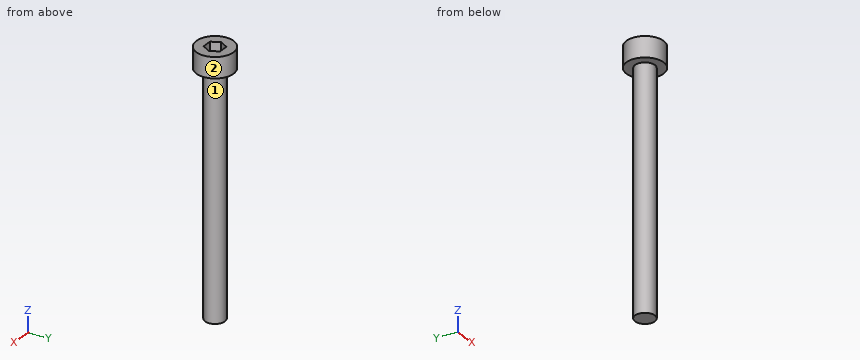
Solid Edge part; units mm, degrees
sketch "Sketch1" plane through (0, 0, 0) normal (0, 0, 1) x (1, 0, 0)
  circle A0 centre (0, 0) radius 2.725
extrude "Protrusion1" add sketch "Sketch1" against normal blind 3
sketch "Sketch2" plane through (0, 0, 0) normal (0, 0, 1) x (1, 0, 0)
  line L0 (-0.7, -1.2124) -> (-1.05, -0.6062)
  line L1 (-1.4, 0) -> (-1.05, -0.6062)
  line L2 (-1.4, 0) -> (-1.05, 0.6062)
  line L3 (-0.7, 1.2124) -> (-1.05, 0.6062)
  line L4 (-0.7, 1.2124) -> (0, 1.2124)
  line L5 (0.7, 1.2124) -> (0, 1.2124)
  line L6 (0.7, 1.2124) -> (1.05, 0.6062)
  line L7 (1.4, 0) -> (1.05, 0.6062)
  line L8 (1.4, 0) -> (1.05, -0.6062)
  line L9 (0.7, -1.2124) -> (1.05, -0.6062)
  line L10 (0.7, -1.2124) -> (0, -1.2124)
  line L11 (-0.7, -1.2124) -> (0, -1.2124)
extrude "ExtrudedCutout_1" cut sketch "Sketch2" against normal blind 1.45
sketch "Sketch3" plane through (0, 0, -3) normal (0, 0, -1) x (1, 0, 0)
  circle A0 centre (0, 0) radius 1.45
extrude "ExtrudedProtrusion_2" add sketch "Sketch3" along normal blind 35
Model file for the job. Use its own axes, mm. Face numbers are marked on the shaded views. A direction names the side the tool comes from. Coordinates: 2 decimals unless noted, no trailing zeros. Write each loop counter-clockwise with the first axis right and the second up, starting at its lowest first coordinate (ties: lowest second). Pieces come first, ordered by that corner, then holes. Notation, with made-up numbers: (55, -27) - (99, -27) arc R32 ccw to (99, 5) - close; hole circle Ø9 at (2, 25.25). An arc over 180 degrees is marked (long way). Write each question's results on one line, items separated by ' | '. Start each with the question number.
1) Cut at D-D (x = -1.95). Write the cut outline in (y, z), then the cut area to 3 significant figures.
2) Cut at A-A (y = -0.4). Write the cut outline in (x, z).
3) 3-axis set-ups, long thin cutter, end or side, ignore diameter. For the marked faces 1 and 2: which of +Z, -Z, +X, -X, +Y, -Y reach the whole face in a straight line?
4) Cut at B-B (x = 0). Write the cut outline in (y, z) (3 decimals).
5) Flat gauge pins, fed straight in: P1, Ø2, axis at y = 0, z = -7, coming from the -X side; P2, Ø1.5, axis at y = -2, z = -30.5, coming from the +X side; P3, Ø3, axis at x = 1, y = -0.5, coming from the +Z side. Where does each tip first touch, or does it go through?
6) Cut at C-C (z = -30.5). Write the cut outline in (x, y), then the cut area to 3 significant figures.
7) Probe line 1 along Y through (x, z) = (0.15, -35); line 2 along Z through (x, y) = (1.7, 1.8); line 3 along Z through (x, y) = (0.55, -1.1). List the from-to ranges inside material, lowest first. Write a range as from..to.
Returned:
1) outline: (-1.9, -3) - (1.9, -3) - (1.9, 0) - (-1.9, 0) - close | area: 11.4 mm^2
2) outline: (-2.7, -3) - (-1.39, -3) - (-1.39, -38) - (1.39, -38) - (1.39, -3) - (2.7, -3) - (2.7, 0) - (1.17, 0) - (1.17, -1.45) - (-1.17, -1.45) - (-1.17, 0) - (-2.7, 0) - close
3) face 1: -Z | face 2: +Z, -Z
4) outline: (-2.725, -3) - (-1.45, -3) - (-1.45, -38) - (1.45, -38) - (1.45, -3) - (2.725, -3) - (2.725, 0) - (1.212, 0) - (1.212, -1.45) - (-1.212, -1.45) - (-1.212, 0) - (-2.725, 0) - close
5) P1: x = -1.45 | P2: x = 0.73 | P3: z = 0
6) outline: circle Ø2.9 at (0, 0) | area: 6.61 mm^2
7) line 1: -1.44..1.44 | line 2: -3..0 | line 3: -38..-1.45
